The model under review builds one solid part; all positions refer to its coordinate system, in mm. Coordinates: 2 decimals unless noted, no trailing zeros. Loops run counter-clockwise (first coordinate to the right, second up) from the corner with the lowest first, then second, coordinate; pieces in that order, holes last. Notation, with made-up numbers: (50.25, 58) - (82.25, 58) arc R15 ccw to (82.25, 71) - close; hole circle Ø2 at (37, -10.75). An arc over 180 degrees is marked (long way). One line per item, written item: value. Start each with the question number.
1. We need section D-D, the plane y = -23. Give the boundary of the cut face in (x, z).
2. We need section C-C, the plane x = 186.69. Give the boundary of the cut face in (y, z).
3. We need section A-A, the plane x = 59.69. Give the boundary of the cut face in (y, z), then the cut area to 3 significant figures.
4. We need section B-B, the plane z = 2.6. Count the separate pieces of the cut face and the enclosed holes in it, then the cut area to 3 significant figures.
5. To check wall thickness, follow line 1 (Y direction, x = 110.5, z = 2.5); line 2 (Y direction, x = 185, z = 1.55); line 3 (Y direction, x = 146, z = 1.8). State the ranges of each line that lie inside material, in increasing order.
Autodesk Inventor part; units mm, degrees
ref_plane "YZ Plane" through (0, 0, 0) normal (1, 0, 0) x (0, 1, 0)
ref_plane "XZ Plane" through (0, 0, 0) normal (0, 1, 0) x (-1, 0, 0)
ref_plane "XY Plane" through (0, 0, 0) normal (0, 0, 1) x (1, 0, 0)
ref_plane "Work Plane1" through (0, 0, 0) normal (0, 0, 1) x (1, 0, 0)
sketch "Sketch1" plane through (0, 0, 0) normal (0, 0, 1) x (1, 0, 0)
  circle A0 centre (59.69, -4.445) radius 1.9304 construction
  circle A1 centre (161.29, -4.445) radius 1.9304 construction
  circle A2 centre (135.89, -4.445) radius 1.9304 construction
  circle A3 centre (34.29, -4.445) radius 1.9304 construction
  circle A4 centre (85.09, -4.445) radius 1.9304 construction
  circle A5 centre (186.69, -4.445) radius 1.9304 construction
  circle A6 centre (110.49, -4.445) radius 1.9304 construction
  circle A7 centre (8.89, -4.445) radius 1.9304 construction
  line L0 (0, 0) -> (0, -8.89) construction
  line L1 (0, -8.89) -> (195.58, -8.89) construction
  line L2 (195.58, 0) -> (195.58, -8.89) construction
  line L3 (0, 0) -> (195.58, 0) construction
  circle A8 centre (254.7602, -6.1683) radius 25.137 construction
  line L4 (0, 0) -> (0, -8.89)
  line L5 (0, -8.89) -> (0, -26.5684)
  line L6 (0, -26.5684) -> (127, -26.5684)
  line L7 (127, -26.5684) -> (223.5038, -13.8825)
  line L8 (223.5038, -13.8825) -> (223.5038, 0)
  line L9 (223.5038, 0) -> (223.5038, 3.81)
  line L10 (223.5038, 3.81) -> (0, 3.81)
  line L11 (0, 3.81) -> (0, 0)
  line L12 (188.7012, -6.3331) -> (188.62, -2.474)
  line L13 (184.6788, -6.3331) -> (184.76, -2.474)
  arc A9 (163.22, -2.474) -> (159.36, -2.474) centre (161.29, -2.5146) ccw
  arc A10 (159.2788, -6.3331) -> (163.3012, -6.3331) centre (161.29, -6.3754) ccw
  line L14 (163.3012, -6.3331) -> (163.22, -2.474)
  line L15 (159.2788, -6.3331) -> (159.36, -2.474)
  arc A11 (137.82, -2.474) -> (133.96, -2.474) centre (135.89, -2.5146) ccw
  line L16 (137.9012, -6.3331) -> (137.82, -2.474)
  line L17 (133.8788, -6.3331) -> (133.96, -2.474)
  arc A12 (108.4788, -6.3331) -> (112.5012, -6.3331) centre (110.49, -6.3754) ccw
  line L18 (112.5012, -6.3331) -> (112.42, -2.474)
  line L19 (108.4788, -6.3331) -> (108.56, -2.474)
  arc A13 (87.02, -2.474) -> (83.16, -2.474) centre (85.09, -2.5146) ccw
  arc A14 (83.0788, -6.3331) -> (87.1012, -6.3331) centre (85.09, -6.3754) ccw
  line L20 (87.1012, -6.3331) -> (87.02, -2.474)
  line L21 (83.0788, -6.3331) -> (83.16, -2.474)
  arc A15 (61.62, -2.474) -> (57.76, -2.474) centre (59.69, -2.5146) ccw
  arc A16 (57.6788, -6.3331) -> (61.7012, -6.3331) centre (59.69, -6.3754) ccw
  line L22 (61.7012, -6.3331) -> (61.62, -2.474)
  line L23 (57.6788, -6.3331) -> (57.76, -2.474)
  arc A17 (36.22, -2.474) -> (32.36, -2.474) centre (34.29, -2.5146) ccw
  arc A18 (32.2788, -6.3331) -> (36.3012, -6.3331) centre (34.29, -6.3754) ccw
  line L24 (36.3012, -6.3331) -> (36.22, -2.474)
  line L25 (32.2788, -6.3331) -> (32.36, -2.474)
  arc A19 (10.82, -2.474) -> (6.96, -2.474) centre (8.89, -2.5146) ccw
  arc A20 (6.8788, -6.3331) -> (10.9012, -6.3331) centre (8.89, -6.3754) ccw
  line L26 (10.9012, -6.3331) -> (10.82, -2.474)
  line L27 (6.8788, -6.3331) -> (6.96, -2.474)
  arc A21 (184.6788, -6.3331) -> (188.7012, -6.3331) centre (186.69, -6.3754) ccw
  arc A22 (188.62, -2.474) -> (184.76, -2.474) centre (186.69, -2.5146) ccw
  arc A23 (133.8788, -6.3331) -> (137.9012, -6.3331) centre (135.89, -6.3754) ccw
  arc A24 (112.42, -2.474) -> (108.56, -2.474) centre (110.49, -2.5146) ccw
  dimension "d0" = 17.6784
  dimension "d1" = 127
  dimension "d2" = 3.81
extrude "Extrusion1" add sketch "Sketch1" along normal blind 3.81
fillet "Fillet1" radius 127 1 edges at (127, -26.5684, 1.905)
properties part number "guide rails"
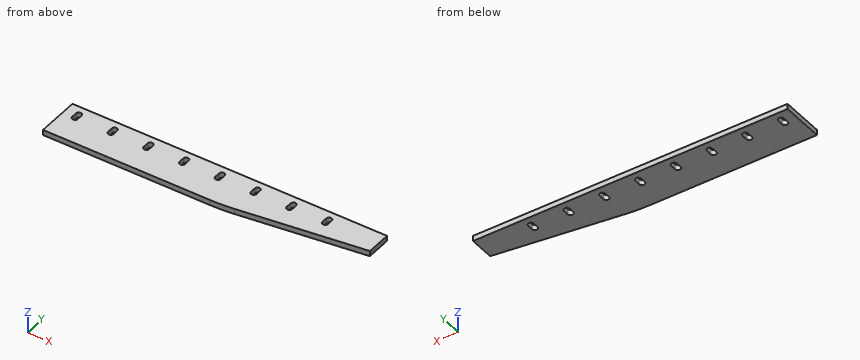
Findings below:
1. outline: (0, 0) - (154.15, 0) - (154.15, 3.81) - (0, 3.81) - close
2. outline: (-18.72, 0) - (-8.39, 0) - (-8.39, 3.81) - (-18.72, 3.81) - close; (-0.58, 0) - (3.81, 0) - (3.81, 3.81) - (-0.58, 3.81) - close
3. outline: (-26.57, 0) - (-8.39, 0) - (-8.39, 3.81) - (-26.57, 3.81) - close; (-0.58, 0) - (3.81, 0) - (3.81, 3.81) - (-0.58, 3.81) - close
3. area: 86.0 mm2
4. separate pieces: 1
4. enclosed holes: 8
4. area: 5,960 mm2
5. line 1: -26.57 to -8.39, -0.58 to 3.81
5. line 2: -18.94 to -7.47, -1.58 to 3.81
5. line 3: -24.07 to 3.81
